The listing builds one solid part. Answer for the finished solid, in the listing's coordinates (mm). Give positions to 0.01 mm unless a question says otherwise; leave off trailing zeros. Loops run counter-clockwise (first coordinate to the right, second up) from the corner with the lowest first, then second, coordinate; pieces in that order, holes last. Notation, with made-up numbers: M -34,-35 L -5,-35 A19 cw -5,-1 Z; hole C 56,0.25 d8. An arc over 180 degrees is marked long. One line per item, written item: value. Start each with the question number.
Q1. Flat-ended cylindrical pins translate along their axes: pin 1 (8 mm diameter, centred on y = 23.5, z = 34, fed in from -X); pin 2 (1.7 mm diameter, centred on x = -20.51, y = 38.89, fed in from -Z); pin 3 (1.5 mm diameter, centred on y = 37, z = 37, fed in from +X); pin 4 (10 mm diameter, centred on x = -22.5, y = 24, fed in from +Z). Find the tip coordinate at first contact, or state that the pin passes through.
Q2. A cutting plane is placed at D-D, the plane y = 37. Determine the outline of the cut face in (x, z), and give its area (3 significant figures).
Q3. A cutting plane is placed at A-A, the plane z = 16.25. State how many separate pieces and enclosed holes the cut face has, and give its area (3 significant figures).
Q4. Consider L1, parallel to Z at x = -17, y = 41.5; L2, parallel to Y at x = -26.5, z = 29.25; L3, parallel to X at y = 35.5, z = 26.75. Determine where each line is inside the solid, lowest interval first.
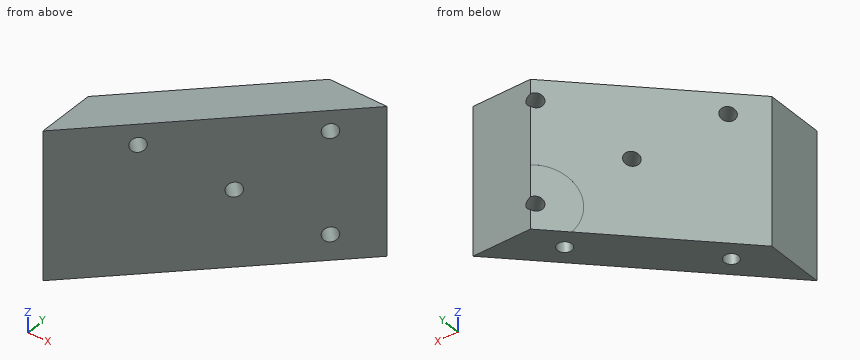
Autodesk Inventor part; units mm, degrees
ref_plane "Work Plane4" through (-34.8055, 8.3289, 16.6138) normal (0.7071068, -0.7071068, 0) x (0.7071068, 0.7071068, 0)
ref_plane "YZ Plane" through (0, 0, 0) normal (1, 0, 0) x (0, 1, 0)
ref_plane "XZ Plane" through (0, 0, 0) normal (0, 1, 0) x (-1, 0, 0)
ref_plane "Work Plane1" through (0, 0, 10) normal (0, 0, 1) x (1, 0, 0)
sketch "Sketch1" plane through (0, 0, 10) normal (0, 0, 1) x (1, 0, 0)
  line L0 (-4.0299, -0.3538) -> (-2.2322, 1.4439) construction
  arc A0 (-1.4439, 2.2322) -> (-2.2322, 1.4439) centre (-0.9299, 0.9299) ccw construction
  line L1 (-1.4439, 2.2322) -> (0.3538, 4.0299) construction
  line L2 (-37.8299, 42.8299) -> (-37.8299, 37.8299) construction
  line L3 (-37.8299, 37.8299) -> (-42.9208, 37.8299) construction
  line L4 (-37.8299, 42.2137) -> (-37.8299, 45.8299) construction
  line L5 (-37.8299, 45.8299) -> (-4.0299, 45.8299) construction
  line L6 (-4.0299, 45.8299) -> (-4.0299, 42.2137) construction
  line L7 (-4.0299, 4.0299) -> (0.3538, 4.0299)
  circle A1 centre (-20.9299, 20.9299) radius 17.5
  line L8 (-20.9299, 58.9723) -> (17.1124, 20.9299) construction
  line L9 (17.1124, 20.9299) -> (-20.9299, -17.1124) construction
  line L10 (-20.9299, -17.1124) -> (-58.9723, 20.9299) construction
  line L11 (-58.9723, 20.9299) -> (-20.9299, 58.9723) construction
  line L12 (-20.9299, 58.9723) -> (-20.9299, -17.1124) construction
  line L13 (17.1124, 20.9299) -> (-58.9723, 20.9299) construction
  line L14 (-20.9299, 58.9723) -> (32.8701, 58.9723) construction
  line L15 (-43.4299, 43.4299) -> (1.5701, 43.4299) construction
  line L16 (1.5701, 43.4299) -> (1.5701, -1.5701) construction
  line L17 (1.5701, -1.5701) -> (-43.4299, -1.5701) construction
  line L18 (-43.4299, -1.5701) -> (-43.4299, 43.4299) construction
  line L19 (-43.4299, 43.4299) -> (1.5701, -1.5701) construction
  line L20 (1.5701, 43.4299) -> (-43.4299, -1.5701) construction
  line L21 (-43.4299, 5.3876) -> (-43.4299, 36.4723)
  line L22 (-43.4299, 36.4723) -> (-36.4723, 43.4299)
  line L23 (-36.4723, 43.4299) -> (-5.3876, 43.4299)
  line L24 (-5.3876, 43.4299) -> (1.5701, 36.4723)
  line L25 (1.5701, 36.4723) -> (1.5701, 5.3876)
  line L26 (1.5701, 5.3876) -> (-5.3876, -1.5701)
  line L27 (-5.3876, -1.5701) -> (-36.4723, -1.5701)
  line L28 (-36.4723, -1.5701) -> (-43.4299, 5.3876)
  line L29 (-4.0299, 42.2137) -> (-37.8299, 42.2137)
  line L30 (-4.0299, -0.3538) -> (-4.0299, 4.0299)
  circle A2 centre (-20.9299, 20.9299) radius 1.4
  line L31 (-10.9299, 10.9299) -> (-30.9299, 10.9299) construction
  line L32 (-30.9299, 10.9299) -> (-30.9299, 30.9299) construction
  line L33 (-30.9299, 30.9299) -> (-10.9299, 30.9299) construction
  line L34 (-10.9299, 30.9299) -> (-10.9299, 10.9299) construction
  line L35 (-10.9299, 10.9299) -> (-30.9299, 30.9299) construction
  line L36 (-30.9299, 10.9299) -> (-10.9299, 30.9299) construction
  circle A3 centre (-30.9299, 30.9299) radius 1.4
  circle A4 centre (-30.9299, 10.9299) radius 1.4
  circle A5 centre (-10.9299, 10.9299) radius 1.4
  line L37 (-45.8299, 37.8299) -> (-42.0723, 37.8299) construction
  line L38 (-42.1723, 37.7299) -> (-45.8299, 37.7299)
  line L39 (-45.8299, 37.7299) -> (-45.8299, 4.1299)
  line L40 (-45.8299, 4.1299) -> (-42.1723, 4.1299)
  line L41 (-42.1723, 4.1299) -> (-42.1723, 37.7299)
  line L42 (-45.8299, 4.0299) -> (-42.0723, 4.0299) construction
  line L43 (-45.8299, 37.8299) -> (-42.0723, 37.8299)
  line L44 (-37.7299, 45.8299) -> (-4.1299, 45.8299)
  line L45 (-4.1299, 45.8299) -> (-4.1299, 42.1723)
  line L46 (-4.1299, 42.1723) -> (-37.7299, 42.1723)
  line L47 (-37.7299, 42.1723) -> (-37.7299, 45.8299)
  line L48 (0.4701, 37.8299) -> (0.4701, 4.0299) construction
  line L49 (0.4701, 4.0299) -> (3.9701, 4.0299) construction
  line L50 (3.9701, 37.8299) -> (3.9701, 4.0299) construction
  line L51 (0.4701, 37.8299) -> (3.9701, 37.8299) construction
  line L52 (-45.8299, -3.9701) -> (-4.0299, -3.9701) construction
  line L53 (0.3124, 37.7299) -> (3.9701, 37.7299)
  line L54 (3.9701, 37.7299) -> (3.9701, 4.1299)
  line L55 (3.9701, 4.1299) -> (0.3124, 4.1299)
  line L56 (0.3124, 4.1299) -> (0.3124, 37.7299)
  line L57 (-4.1713, -0.3538) -> (-37.7299, -0.3538)
  line L58 (-37.7299, -0.3538) -> (-37.7299, -3.9701)
  line L59 (-37.7299, -3.9701) -> (-4.1713, -3.9701)
  line L60 (-4.1713, -3.9701) -> (-4.1713, -0.3538)
  point P0 (-37.8299, 4.0299)
  dimension "d18" = 53.8
  dimension "d19" = 45
  dimension "d20" = 53.8
  dimension "d21" = 45
  dimension "d22" = 45
  dimension "d30" = 20
  dimension "d31" = 20
  dimension "d32" = 2.8
  dimension "d33" = 2.8
  dimension "d34" = 2.8
  dimension "d35" = 2.8
  dimension "d36" = 0.1
  dimension "d37" = 0.1
  dimension "d38" = 0.1
  dimension "d39" = 0.1
extrude "Extrusion1" add sketch "Sketch1" along normal blind 5 contours L30 L26 L57 L28 L41 L22 L46 L24 L56 L7 | L7 L26 L30 | L56 L24 L25 L26 | L26 L25 L24 L53 L54 L55 | L60 L59 L58 L57 L28 L27 L26 | L26 L27 L28 L57 | L46 L22 L29 L24 | L24 L29 L45 | L40 L39 L38 L22 L21 L28 | L28 L21 L22 L41 | L29 L22 L23 L24 | L24 L23 L22 L29 L47 L44 L45 | L47 L29 L22 | A1 | A2 | A3 | A4 | A5
sketch "Sketch4" plane through (0, 0, 15) normal (0, 0, 1) x (1, 0, 0)
  line L0 (-37.7299, 42.1723) -> (-42.1723, 37.7299)
  line L1 (-42.1723, 37.7299) -> (-45.8299, 37.7299)
  line L2 (-45.8299, 37.7299) -> (-45.8299, 4.1299)
  line L3 (-45.8299, 4.1299) -> (-42.1723, 4.1299)
  line L4 (-42.1723, 4.1299) -> (-37.6885, -0.3538)
  line L5 (-37.6885, -0.3538) -> (-37.7299, -0.3538)
  line L6 (-37.7299, -0.3538) -> (-37.7299, -3.9701)
  line L7 (-37.7299, -3.9701) -> (-4.1713, -3.9701)
  line L8 (-4.1713, -3.9701) -> (-4.1713, -0.3538)
  line L9 (-4.1713, -0.3538) -> (0.3124, 4.1299)
  line L10 (0.3124, 4.1299) -> (3.9701, 4.1299)
  line L11 (3.9701, 4.1299) -> (3.9701, 37.7299)
  line L12 (3.9701, 37.7299) -> (0.3124, 37.7299)
  line L13 (0.3124, 37.7299) -> (-4.1299, 42.1723)
  line L14 (-4.1299, 42.1723) -> (-4.1299, 45.8299)
  line L15 (-4.1299, 45.8299) -> (-37.7299, 45.8299)
  line L16 (-37.7299, 45.8299) -> (-37.7299, 42.1723)
  line L17 (-45.8299, 37.7299) -> (-45.8299, 4.1299)
  line L18 (-45.8299, 7.911) -> (-7.911, 45.8299)
  line L19 (-45.8299, 7.911) -> (7.7955, 7.911) construction
  line L20 (-7.911, 45.8299) -> (-19.2247, 45.8299)
  line L21 (-4.1299, 45.8299) -> (-37.7299, 45.8299)
  line L22 (-19.2247, 45.8299) -> (-45.8299, 19.2247)
  line L23 (-45.8299, 7.911) -> (-45.8299, 19.2247)
  circle A0 centre (-40.9299, 0.9299) radius 1.1933
  circle A1 centre (-0.9299, 40.9299) radius 1.4
  line L24 (-40.9299, 0.9299) -> (-0.9299, 40.9299)
  line L25 (0.3124, 37.7299) -> (-4.1299, 42.1723)
  point P0 (0, 0)
  dimension "d40" = 45
  dimension "d41" = 8
extrude "Extrusion4" add sketch "Sketch4" along normal blind 28 contours L15 L18 L2 L22
sketch "Sketch5" plane through (-45.8299, 19.2247, 15) normal (-0.7071068, 0.7071068, 0) x (-0.7071068, -0.7071068, 0)
  line L0 (0, 0) -> (-37.6254, 0)
  line L1 (0, 0) -> (0, 28)
  line L2 (-37.6254, 28) -> (0, 28)
  line L3 (-37.6254, 0) -> (-37.6254, 28)
  circle A0 centre (-18.8127, 9.1873) radius 18.8127
  line L4 (-6.8127, 24) -> (-36.8127, 24) construction
  line L5 (-36.8127, 24) -> (-36.8127, 4) construction
  line L6 (-36.8127, 4) -> (-6.8127, 4) construction
  line L7 (-6.8127, 4) -> (-6.8127, 24) construction
  line L8 (-6.8127, 24) -> (-36.8127, 4) construction
  line L9 (-36.8127, 24) -> (-6.8127, 4) construction
  point P0 (-18.8127, -15)
  point P1 (-21.8127, 14)
  dimension "d44" = 30
  dimension "d45" = 20
hole "Hole1" at (-19.7994, 45.2552, 39) at (-19.7994, 45.2552, 19) at (-41.0126, 24.042, 39) at (-30.406, 34.6486, 29) direction (0.7071068, -0.7071068, 0) diameter 2.9 depth 12
sketch "Sketch6" plane through (-37.7299, -3.9701, 10) normal (0, -1, 0) x (1, 0, 0)
  circle A0 centre (-3.2, 36.9) radius 1.45
  circle A1 centre (36.8, 36.9) radius 1.45
  line L0 (-6.1, 0) -> (-6.1, 39.8)
  line L1 (-0.1, 0) -> (-6.1, 0)
  line L2 (-0.1, 33.8) -> (-0.1, 0)
  line L3 (33.7, 33.8) -> (-0.1, 33.8)
  line L4 (33.7, 33.8) -> (33.7, 0)
  line L5 (39.7, 0) -> (33.7, 0)
  line L6 (39.7, 39.8) -> (39.7, 0)
  line L7 (-6.1, 39.8) -> (39.7, 39.8)
  circle A2 centre (16.8, 16.9) radius 16.9
  circle A3 centre (16.8, 16.9) radius 14.9
  line L8 (-0.1, 16.9) -> (-0.1, 0)
  line L9 (0, 0) -> (33.5586, 0)
  line L10 (0.0414, 0) -> (-4.4423, 0)
  line L11 (33.5586, 0) -> (0.0414, 0)
  line L12 (33.7, 16.9) -> (33.5586, 0)
  point P0 (37.7299, -10)
  dimension "d53" = 2
extrude "Extrusion5" cut sketch "Sketch6" against normal up to surface contours A3 surface through (-45.8299, 7.911, 15) normal (0.7071068, -0.7071068, 0)
ref_plane "Work Plane3" through (3.9701, 45.8299, 26) normal (1, 0, 0) x (0, -1, 0)
sketch "Sketch7" plane through (3.9701, 45.8299, 26) normal (1, 0, 0) x (0, -1, 0)
  line L0 (41.8, -17.8) -> (41.8, 16)
  line L1 (8, -17.8) -> (41.8, -17.8)
  line L2 (8, -17.8) -> (8, 16)
  circle A0 centre (24.9, -0.9) radius 16.9
  circle A1 centre (24.9, -0.9) radius 14.9
  point P0 (45.8299, 26)
  dimension "d56" = 2
ref_plane "Work Plane4" through (-34.8055, 8.3289, 16.6138) normal (0.7071068, -0.7071068, 0) x (0.7071068, 0.7071068, 0)
extrude "Extrusion6" cut sketch "Sketch7" against normal up to surface contours A1 surface through (-45.8299, 7.911, 15) normal (0.7071068, -0.7071068, 0)
sketch "Sketch8" plane through (-45.8299, 19.2247, 15) normal (-0.7071068, 0.7071068, 0) x (-0.7071068, -0.7071068, 0)
  arc A0 (-37.6254, 2.7992) -> (-37.6254, 5.2008) centre (-36.8127, 4) ccw
  circle A1 centre (-36.8127, 4) radius 7.5
  point P0 (-18.8127, -15)
  dimension "d59" = 15
extrude "Extrusion7" cut sketch "Sketch8" along normal blind 10
sketch "Sketch9" plane through (0, 0, 10) normal (0, 0, -1) x (-1, 0, 0)
  line L0 (45.8299, 19.2247) -> (24.2855, 40.7692)
  line L1 (41.7776, 11.9633) -> (26.8705, 26.8705)
  line L2 (26.8705, 26.8705) -> (11.9633, 41.7776)
  line L3 (19.2247, 45.8299) -> (24.2855, 40.7692)
  line L4 (7.911, 45.8299) -> (11.9633, 41.7776)
  line L5 (41.7776, 11.9633) -> (45.8299, 7.911)
  line L6 (15.1679, 38.5731) -> (20.8247, 44.2299)
  line L7 (13.1172, 40.6237) -> (18.3235, 45.8299)
  line L8 (34.3304, 19.4105) -> (39.9873, 25.0673)
  line L9 (36.3811, 17.3599) -> (42.0379, 23.0167)
  circle A0 centre (20.5065, 38.8913) radius 1.4
  line L10 (25.7745, 27.9665) -> (31.4313, 33.6233)
  line L11 (31.4313, 33.6233) -> (25.7745, 27.9665)
  line L12 (26.8705, 26.8705) -> (32.5273, 32.5273)
  circle A1 centre (38.8913, 20.5065) radius 1.4
  point P0 (0, 0)
  point P1 (34.7528, 24.7491)
  dimension "d62" = 2.8
hole "Hole2" at (-20.5065, 38.8913, 10) at (-38.8913, 20.5065, 10) direction (0, 0, 1) diameter 2.8 depth 12 counterbore diameter 5.5 counterbore depth 3
sketch "Sketch11" plane through (0, 0, 43) normal (0, 0, 1) x (1, 0, 0)
  line L0 (-7.911, 45.8299) -> (-19.2247, 45.8299)
  line L1 (-19.2247, 45.8299) -> (-45.8299, 19.2247)
  line L2 (-45.8299, 19.2247) -> (-45.8299, 7.911)
  line L3 (-45.8299, 7.911) -> (-7.911, 45.8299)
  line L4 (-45.8299, 37.7299) -> (-45.8299, 19.2247)
  line L5 (-42.1723, 37.7299) -> (-45.8299, 37.7299)
  line L6 (-37.7299, 42.1723) -> (-42.1723, 37.7299)
  line L7 (-37.7299, 45.8299) -> (-37.7299, 42.1723)
  line L8 (-29.3463, 45.8299) -> (-37.7299, 45.8299)
  line L9 (-29.3463, 45.8299) -> (-19.2247, 45.8299)
  line L10 (-4.1299, 45.8299) -> (-7.911, 45.8299)
  line L11 (-4.1299, 42.1723) -> (-4.1299, 45.8299)
  line L12 (0.3124, 37.7299) -> (-4.1299, 42.1723)
  line L13 (3.9701, 37.7299) -> (0.3124, 37.7299)
  line L14 (3.9701, 29.8965) -> (3.9701, 11.9633)
  line L15 (3.9701, 29.8965) -> (3.9701, 37.7299)
  line L16 (-11.9633, -3.9701) -> (-4.1713, -3.9701)
  line L17 (-4.1713, -3.9701) -> (-4.1713, -0.3538)
  line L18 (-4.1713, -0.3538) -> (0.3124, 4.1299)
  line L19 (0.3124, 4.1299) -> (3.9701, 4.1299)
  line L20 (3.9701, 4.1299) -> (3.9701, 11.9633)
  line L21 (-11.9633, -3.9701) -> (-29.8965, -3.9701)
  line L22 (-37.7299, -3.9701) -> (-29.8965, -3.9701)
  line L23 (-37.7299, -0.3538) -> (-37.7299, -3.9701)
  line L24 (-45.8299, 7.911) -> (-7.911, 45.8299)
  line L25 (-45.8299, 7.911) -> (-7.911, 45.8299)
  line L26 (-45.8299, 7.911) -> (-45.8299, 4.1299)
  line L27 (-45.8299, 4.1299) -> (-42.1723, 4.1299)
  line L28 (-37.6885, -0.3538) -> (-37.7299, -0.3538)
  line L29 (-42.1723, 4.1299) -> (-37.6885, -0.3538)
  point P0 (0, 0)
extrude "Extrusion8" cut sketch "Sketch11" against normal through all contours L10 L11 L12 L13 L15 L14 L20 L19 L18 L17 L16 L21 L22 L23 L28 L29 L27 L26 L3 | L1 L4 L5 L6 L7 L8 L9
sketch "Sketch12" plane through (-45.8299, 19.2247, 10) normal (-0.7071068, 0.7071068, 0) x (-0.7071068, -0.7071068, 0)
  line L0 (-45.6254, 33) -> (-45.6254, 0)
  line L1 (8, 0) -> (8, 33)
  line L2 (-45.6254, 0) -> (8, 0)
  line L3 (8, 0) -> (8, 4)
  line L4 (8, 4) -> (-45.6254, 4)
  line L5 (-45.6254, 4) -> (-45.6254, 0)
  point P0 (-18.8127, -10)
  point P1 (45.6254, -4)
  point P2 (45.6254, -5)
  point P3 (-8, -5)
  point P4 (-8, -4)
  dimension "d73" = 4
extrude "Extrusion9" cut sketch "Sketch12" against normal blind 29
properties part number "20_Cube_Insert_Kinematic_Mirrormount_45_base_part2"
Answer block:
1. pin 1: x = -45.55
1. pin 2: z = 22
1. pin 3: x = -15.99
1. pin 4: through
2. outline: M -28.05,14 L -16.74,14 L -16.74,43 L -28.05,43 Z
2. area: 328 mm^2
3. separate pieces: 1
3. enclosed holes: 2
3. area: 353 mm^2
4. L1: 14 to 17.72, 20.28 to 37.72, 40.28 to 43
4. L2: 27.24 to 28.72, 32.76 to 38.55
4. L3: -29.55 to -18.24
